Here's how the part is built. I have some questions about the finished solid (model axes, mm). A direction names the side the tool comes from. Give positions to 0.01 mm unless a question says otherwise; leave off trailing zeros. Write each loop counter-clockwise with the first axis right and the second up, starting at its lowest first coordinate (ties: lowest second). Pieces come first, ordered by that corner, then holes. Notation, with made-up numbers: M 26.25,67.5 L 52.25,67.5 A25 ccw 52.25,106.5 Z; hole C 54.25,88.25 d5. An arc over 180 degrees is marked long. Answer as CSV lines item,"result". Start each with the question number.
Q1. For pin 1 (0.5 mm diameter, centred on x = 2, y = 2, fed in from +Z); pin 2 (1.9 mm diameter, centred on x = -1, y = 10, fed in from -Z); pin 3 (1 mm diameter, centred on x = -2, y = 2.5, fed in from -Z), each with a flat end and sliding along its axis, tell me the tip position at first contact or that it passes through.
Q2. Suppose I cut it at C-C (x = -2). Write out the boundary of the cut face in (y, z).
Q3. If I drill on line 1 along Y through (x, z) = (0, 0.25); line 2 along Y through (x, z) = (0, -3.7); line 3 along X through (y, z) = (6.5, 1.5), over which ranges is the centre line in solid material (lowest first)?
Q4. Suppose I cut it at B-B (z = 0). Write out the boundary of the cut face in (x, y).
Q5. Suppose I cut it at A-A (y = 8.5). Write out the boundary of the cut face in (x, z).
Q6. Thinking about a two-plate mould opening in Z: for faces 1 (the cylindrical face through (-3.1, 3.4, 0)), 2 (the cylindrical face through (1.29, 10.524, 0.042)), 3 (the flat face through (1, 6, -3)), 4 (the flat face through (0.84, 2, -2)), which applies, +Z half, -Z half, draft (parallel to the pull), parting line (faces both ways), or undercut?
Q7. On a 3-axis mill with a long thin cutter (end or side, diameter ignored), from which of +Z, -Z, +X, -X, +Y, -Y can I reach the whole of each face in a straight line? I mean faces 5 (the flat face through (-0.84, 2, -2)), 6 (the cylindrical face through (1.43, 5.75, 3.51)), 7 (the cylindrical face through (1.9, 2.5, 1.9)), 8 (the cylindrical face through (1.43, 5.75, -3.51)). Say none if no direction works.
```python
from build123d import *

# Parameters (mm, degrees)
BOSS_EXTRUDE1_DEPTH = 7
FILLET1_R           = 6.2
FILLET2_R           = 6.2
FILLET3_R           = 6.2
FILLET4_R           = 6.2
CUT_EXTRUDE1_DEPTH  = 5
SKETCH5_R           = 3.5
BOSS_EXTRUDE2_DEPTH = 4
SKETCH9_R           = 2.4
CUT_EXTRUDE2_DEPTH  = 15.840822238
SKETCH10_R          = 3.1
CUT_EXTRUDE3_DEPTH  = 1
FILLET5_R           = 0.4
FILLET6_R           = 0.4
FILLET7_R           = 0.4
FILLET8_R           = 0.4
FILLET9_R           = 0.1
FILLET10_R          = 0.1
FILLET11_R          = 0.1
FILLET12_R          = 0.1
FILLET13_R          = 0.1
FILLET14_R          = 0.1
FILLET15_R          = 0.1
FILLET16_R          = 0.1


with BuildPart() as part:
    # Sketch2 → Boss-Extrude1 (new body)
    with BuildSketch(Plane(origin=(0, 0, 0), x_dir=(1, 0, 0), z_dir=(0, 1, 0))):
        with BuildLine():
            Line((-1.085, -1.085), (-1.085, -2.903924069))
            ThreePointArc((-1.085, -2.903924069), (0, -3.1), (1.085, -2.903924069))
            Line((1.085, -2.903924069), (1.085, -1.085))
            Line((1.085, -1.085), (2.903924069, -1.085))
            ThreePointArc((2.903924069, -1.085), (3.1, 0), (2.903924069, 1.085))
            Line((2.903924069, 1.085), (1.085, 1.085))
            Line((1.085, 1.085), (1.085, 2.903924069))
            ThreePointArc((1.085, 2.903924069), (0, 3.1), (-1.085, 2.903924069))
            Line((-1.085, 2.903924069), (-1.085, 1.085))
            Line((-1.085, 1.085), (-2.903924069, 1.085))
            ThreePointArc((-2.903924069, 1.085), (-3.1, 0), (-2.903924069, -1.085))
            Line((-2.903924069, -1.085), (-1.085, -1.085))
        make_face()
    extrude(amount=BOSS_EXTRUDE1_DEPTH)

    # Fillet1
    # the kernel refuses this fillet: 6.2 mm, written as the material it adds along each edge
    with BuildSketch(Plane(origin=(-1.085, 0, -1.085), x_dir=(0, 0, -1), z_dir=(0, 1, 0))) as fillet1_piece_1:
        with BuildLine():
            CenterArc((5.198154004, 5.198154004), FILLET1_R, 213.027198012, 23.945603977)
            Line((0, 1.818924069), (0, 0))
            Line((0, 0), (1.818924069, 0))
        make_face()
    extrude(amount=7)

    # Fillet2
    # the kernel refuses this fillet: 6.2 mm, written as the material it adds along each edge
    with BuildSketch(Plane(origin=(1.085, 0, -1.085), x_dir=(0, 0, -1), z_dir=(0, 1, 0))) as fillet2_piece_1:
        with BuildLine():
            CenterArc((5.198154004, -5.198154004), FILLET2_R, 123.027198012, 23.945603977)
            Line((0, -1.818924069), (0, 0))
            Line((0, 0), (1.818924069, 0))
        make_face()
    extrude(amount=7)

    # Fillet3
    # the kernel refuses this fillet: 6.2 mm, written as the material it adds along each edge
    with BuildSketch(Plane(origin=(1.085, 0, 1.085), x_dir=(1, 0, 0), z_dir=(0, 1, 0))) as fillet3_piece_1:
        with BuildLine():
            CenterArc((5.198154004, -5.198154004), FILLET3_R, 123.027198012, 23.945603977)
            Line((0, -1.818924069), (0, 0))
            Line((0, 0), (1.818924069, 0))
        make_face()
    extrude(amount=7)

    # Fillet4
    # the kernel refuses this fillet: 6.2 mm, written as the material it adds along each edge
    with BuildSketch(Plane(origin=(-1.085, 0, 1.085), x_dir=(0, 0, 1), z_dir=(0, 1, 0))) as fillet4_piece_1:
        with BuildLine():
            CenterArc((5.198154004, -5.198154004), FILLET4_R, 123.027198012, 23.945603977)
            Line((0, -1.818924069), (0, 0))
            Line((0, 0), (1.818924069, 0))
        make_face()
    extrude(amount=7)

    # Sketch4 → Cut-Extrude1 (cut)
    with BuildSketch(Plane.XZ):
        with BuildLine():
            Line((0.84, 0.84), (0.84, 2.248199279))
            ThreePointArc((0.84, 2.248199279), (0, 2.4), (-0.84, 2.248199279))
            Line((-0.84, 2.248199279), (-0.84, 0.84))
            Line((-0.84, 0.84), (-2.248199279, 0.84))
            ThreePointArc((-2.248199279, 0.84), (-2.4, 0), (-2.248199279, -0.84))
            Line((-2.248199279, -0.84), (-0.84, -0.84))
            Line((-0.84, -0.84), (-0.84, -2.248199279))
            ThreePointArc((-0.84, -2.248199279), (0, -2.4), (0.84, -2.248199279))
            Line((0.84, -2.248199279), (0.84, -0.84))
            Line((0.84, -0.84), (2.248199279, -0.84))
            ThreePointArc((2.248199279, -0.84), (2.4, 0), (2.248199279, 0.84))
            Line((2.248199279, 0.84), (0.84, 0.84))
        make_face()
    extrude(amount=-CUT_EXTRUDE1_DEPTH, mode=Mode.SUBTRACT)

    # Sketch5 → Boss-Extrude2 (add, symmetric)
    with BuildSketch(Plane.XY):
        with Locations((0, 8.5)):
            Circle(SKETCH5_R)
    extrude(amount=BOSS_EXTRUDE2_DEPTH, both=True)

    # Sketch9 → Cut-Extrude2 (cut, through all)
    with BuildSketch(Plane.XY.offset(4)):
        with Locations((0, 8.5)):
            Circle(SKETCH9_R)
    extrude(amount=-CUT_EXTRUDE2_DEPTH, mode=Mode.SUBTRACT)

    # Sketch10 → Cut-Extrude3 (cut)
    with BuildSketch(Plane.XY.offset(4)):
        with Locations((0, 8.5)):
            Circle(SKETCH10_R)
    cut_extrude3 = extrude(amount=-CUT_EXTRUDE3_DEPTH, mode=Mode.SUBTRACT)

    # Mirror1: Cut-Extrude3 across plane
    add(cut_extrude3.mirror(Plane.XY), mode=Mode.SUBTRACT)

    # Fillet5
    fillet5_edges = [part.edges().sort_by_distance(p)[0] for p in [
        (0.84, 2.5, 0.84),
    ]]
    fillet(fillet5_edges, radius=FILLET5_R)

    # Fillet6
    fillet6_edges = [part.edges().sort_by_distance(p)[0] for p in [
        (-0.84, 2.5, 0.84),
    ]]
    fillet(fillet6_edges, radius=FILLET6_R)

    # Fillet7
    fillet7_edges = [part.edges().sort_by_distance(p)[0] for p in [
        (-0.84, 2.5, -0.84),
    ]]
    fillet(fillet7_edges, radius=FILLET7_R)

    # Fillet8
    fillet8_edges = [part.edges().sort_by_distance(p)[0] for p in [
        (0.84, 2.5, -0.84),
    ]]
    fillet(fillet8_edges, radius=FILLET8_R)

    # Fillet9
    fillet9_edges = [part.edges().sort_by_distance(p)[0] for p in [
        (-0.84, 2.5, 2.248199279),
    ]]
    fillet(fillet9_edges, radius=FILLET9_R)

    # Fillet10
    fillet10_edges = [part.edges().sort_by_distance(p)[0] for p in [
        (0.84, 2.5, 2.248199279),
    ]]
    fillet(fillet10_edges, radius=FILLET10_R)

    # Fillet11
    fillet11_edges = [part.edges().sort_by_distance(p)[0] for p in [
        (-2.248199279, 2.5, -0.84),
    ]]
    fillet(fillet11_edges, radius=FILLET11_R)

    # Fillet12
    fillet12_edges = [part.edges().sort_by_distance(p)[0] for p in [
        (-2.248199279, 2.5, 0.84),
    ]]
    fillet(fillet12_edges, radius=FILLET12_R)

    # Fillet13
    fillet13_edges = [part.edges().sort_by_distance(p)[0] for p in [
        (2.248199279, 2.5, 0.84),
    ]]
    fillet(fillet13_edges, radius=FILLET13_R)

    # Fillet14
    fillet14_edges = [part.edges().sort_by_distance(p)[0] for p in [
        (2.248199279, 2.5, -0.84),
    ]]
    fillet(fillet14_edges, radius=FILLET14_R)

    # Fillet15
    fillet15_edges = [part.edges().sort_by_distance(p)[0] for p in [
        (-0.84, 2.5, -2.248199279),
    ]]
    fillet(fillet15_edges, radius=FILLET15_R)

    # Fillet16
    fillet16_edges = [part.edges().sort_by_distance(p)[0] for p in [
        (0.84, 2.5, -2.248199279),
    ]]
    fillet(fillet16_edges, radius=FILLET16_R)


solid = part.part
```
Resolved:
1,pin 1,"z = 2.05"
1,pin 2,"z = -3"
1,pin 3,"z = -2.34"
2,outline,"M 0,-1.8 L 5.63,-1.8 L 5.63,-4 L 6.13,-4 L 6.13,-3 L 7.17,-3 L 7.17,3 L 6.13,3 L 6.13,4 L 5.63,4 L 5.63,1.8 L 0,1.8 L 0,0.84 L 5,0.84 L 5,-0.84 L 0,-0.84 Z; M 9.83,-3 L 10.87,-3 L 10.87,-4 L 11.37,-4 L 11.37,4 L 10.87,4 L 10.87,3 L 9.83,3 Z"
3,line 1,"5 to 6.1, 10.9 to 12"
3,line 2,"5 to 5.4, 11.6 to 12"
3,line 3,"-2.87 to -1.33, 1.33 to 2.87"
4,outline,"M -3.1,0 L -2.4,0 L -2.4,5 L 2.4,5 L 2.4,0 L 3.1,0 L 3.1,6.88 A3.5 ccw long -3.1,6.88 Z; hole C 0,8.5 d4.8"
5,outline,"M -3.5,-4 L -3.1,-4 L -3.1,-3 L -2.4,-3 L -2.4,3 L -3.1,3 L -3.1,4 L -3.5,4 Z; M 2.4,-3 L 3.1,-3 L 3.1,-4 L 3.5,-4 L 3.5,4 L 3.1,4 L 3.1,3 L 2.4,3 Z"
6,face 1,"parting line"
6,face 2,"draft"
6,face 3,"-Z half"
6,face 4,"undercut"
7,face 5,"-Y"
7,face 6,"+Z"
7,face 7,"+Z, +X, -Y"
7,face 8,"-Z"
